Source: CAD feature listing. Evaluate the final solid. Frame: model axes, mm. A direction names the side the tool comes from. Coordinates: 2 decimals unless noted, no trailing zeros. Write each loop counter-clockwise with the first axis right and the second up, starting at its lowest first coordinate (ties: lowest second). Pieces come first, ordered by that corner, then holes. Notation, with made-up numbers: (58, -13) - (110, -13) arc R9 cw to (110, 2) - close; hole circle Ø3 at (62, 50.25). An arc over 180 degrees is marked (long way). One line per question, with ' | ' between items. Start each with the question number.
Q1. Cut plane B-B, the plane x = 1.75. Return loops of the section in (y, z), plus the area to 3 significant figures.
Q2. Cut plane C-C, the plane z = -3. Return loops of the section in (x, y) (3 decimals).
Q3. Line query: line 1 (X direction, y = -3.25, z = -8) (3 decimals); line 2 (Z direction, x = 4, y = -1.5); line 3 (Z direction, x = 0.25, y = -6.25). Output: solid intervals per line, ascending.
Q4. Contact query for flat-ended pins moving along their axis: P1, Ø4, axis at y = -5, z = -11.5, coming from the -X side; P2, Ø2.5, axis at x = -8, y = -3.5, coming from the -Z side; P3, Ø1, axis at x = -2.5, y = -6, coming from the +Z side. Output: stop coordinate, or through.
Q5. Draft query along Z for faces 5 (the face through (2, 0, -7)), 6 (the face through (3.69, -3.757, -24.435)), 7 (the face through (-5, -4, 0)). Return one class per face: +Z half, -Z half, draft (parallel to the pull), parting line (faces both ways), or undercut.
Q6. Access query for faces 1 (the face through (-10.561, -4, -19)), 2 (the face through (3.002, -4, 6)), 3 (the face through (-8, -4, -17.78)), 4 (the face through (-2.68, -3.76, -20.52)). Directions: +Z, -Z, +X, -X, +Y, -Y. A direction counts if a zero-diameter tool reaches every point of the face in a straight line with its end or side. Return the directions, or none.
Q7. Cut plane D-D, the plane x = 8.25. Return loops of the section in (y, z).
```python
from build123d import *

# Parameters (mm, degrees)
F0_R     = 1.905
F1_DEPTH = 7.62


with BuildPart() as f1:
    # F0 (on Front) → F1 (new body)
    with BuildSketch(Plane.XZ):
        with BuildLine():
            Line((1.1841486596, 5.08), (-10.795, 5.08))
            Line((-10.795, 5.08), (-10.795, 0))
            Line((-10.795, 0), (0, 0))
            Line((0, 0), (0, -17.78))
            ThreePointArc((0, -17.78), (-2.7403535787, -20.5203535787), (-5.4807071574, -17.78))
            Line((-5.4807071574, -17.78), (-10.5607071574, -17.78))
            Line((-10.5607071574, -17.78), (-10.5607071574, -20.2195488962))
            ThreePointArc((-10.5607071574, -20.2195488962), (-7.6870708125, -23.955222101), (-3.3948952839, -25.9020835155))
            ThreePointArc((-3.3948952839, -25.9020835155), (3.7738885263, -24.3699633295), (6.985, -17.78))
            Line((6.985, -17.78), (6.985, 0))
            Line((6.985, 0), (14.605, 0))
            Line((14.605, 0), (14.605, 5.08))
            Line((14.605, 5.08), (3.0016307719, 5.08))
            Line((3.0016307719, 5.08), (1.1841486596, 5.08))
        make_face()
        with BuildLine():
            Line((1.1841486596, 7.7244357235), (1.1841486596, 5.08))
            Line((1.1841486596, 5.08), (3.0016307719, 5.08))
            Line((3.0016307719, 5.08), (3.0016307719, 7.7244357235))
            Line((3.0016307719, 7.7244357235), (2.6258513404, 7.7244357235))
            ThreePointArc((2.6258513404, 7.7244357235), (1.905, 7.62), (1.1841486596, 7.7244357235))
        make_face()
        with BuildLine():
            Line((2.6258513404, 7.7244357235), (1.1841486596, 7.7244357235))
            ThreePointArc((1.1841486596, 7.7244357235), (1.905, 7.62), (2.6258513404, 7.7244357235))
        make_face()
        with BuildLine():
            ThreePointArc((4.445, 10.16), (0.3850267115, 12.1950138089), (1.1841486596, 7.7244357235))
            Line((1.1841486596, 7.7244357235), (2.6258513404, 7.7244357235))
            ThreePointArc((2.6258513404, 7.7244357235), (3.9400138089, 8.6400267115), (4.445, 10.16))
        make_face()
        with Locations((1.905, 10.16)):
            Circle(F0_R, mode=Mode.SUBTRACT)
    extrude(amount=F1_DEPTH)


solid = f1.part
```
Reply:
1) outline: (-7.62, -25.54) - (0, -25.54) - (0, 8.26) - (-7.62, 8.26) - close; (-7.62, 12.06) - (0, 12.06) - (0, 12.7) - (-7.62, 12.7) - close | area: 262 mm^2
2) outline: (0, -7.62) - (6.985, -7.62) - (6.985, 0) - (0, 0) - close
3) line 1: x = 0 to 6.985 | line 2: z = -24.19 to 5.08, 8.72 to 11.6 | line 3: z = -25.99 to 5.08, 8.23 to 9.22, 11.1 to 12.09
4) P1: stops at x = 0 | P2: stops at z = -24.61 | P3: stops at z = 5.08
5) face 5: draft | face 6: -Z half | face 7: undercut
6) face 1: -Z, -X, +Y, -Y | face 2: +X, +Y, -Y | face 3: -X, +Y, -Y | face 4: +Y, -Y
7) outline: (-7.62, 0) - (0, 0) - (0, 5.08) - (-7.62, 5.08) - close
